Design review of the part built by this model. Coordinates are the model's own, in mm. A direction names the side the tool comes from. Coordinates: 2 decimals unless noted, no trailing zeros. Loops run counter-clockwise (first coordinate to the right, second up) from the corner with the lowest first, then second, coordinate; pieces in that order, holes last. Notation, with made-up numbers: (8, 25) -> (15, 25) arc R6 ccw to (15, 36) -> close; hole circle Ø2 at (71.25, -30). An arc over 180 degrees is marked (long way). Use one line per item in the form item = value. Start each with the question number.
1. For pin 1 (16.5 mm diameter, centred on x = 162.54, z = 38.1, fed in from -Y); pin 2 (4 mm diameter, centred on y = 28.5, z = 74, fed in from -X); pin 3 (2.5 mm diameter, centred on y = 36.5, z = 74.5, fed in from +X), all flat-tipped, find the tip position at first contact; note any pin that passes through.
2. Wall thickness on line 1 (Z direction, x = 19.05, y = 2.55); line 2 (X direction, y = 57, z = 25); line 3 (Y direction, x = 169.5, z = 46.5) (1 decimal): over which ranges is each line inside the solid? List them lowest first. Write a range as from..to.
3. Consider section B-B (y = 13.5). State the section outline as (x, z) points.
4. Consider section C-C (z = 25.4). State the section outline as (x, y) points (1 decimal).
5. Consider section D-D (x = 112). State the section outline as (y, z) points (1 decimal), then the cut area to 3 significant figures.
6. Machinability: for faces 1 (the face through (119, 30, 4.763)), 2 (the face through (14.292, 57.91, 25.609)), 3 (the face through (102.763, 30, 74)), 4 (the face through (135.793, 30, 2)), which of the approach directions +Z, -Z, +X, -X, +Y, -Y give a long, thin tool a straight path to every point of the face, cutting with its end or side? Answer none if there is none.
7. The part is to be moulded in two halves that separate along Y. For faces 5 (the face through (157.5, 57.91, 34.236)), 6 (the face through (100, 55.562, 38)), 7 (the face through (100, 60.325, 39)), say which applies: released by +Y, released by -Y, zero draft, split by the parting line, or undercut.
8. Consider section A-A (z = 38.1). State the section outline as (x, y) points (1 decimal), then the cut area to 3 significant figures.
from build123d import *

# Parameters (mm, degrees)
F0_W     = 203.2
F0_H     = 76.2
F0_R     = 4.7625
F0_R_2   = 6.35
F1_DEPTH = 60.325
F3_W     = 102.7627293737
F3_H     = 50.8
F4_DEPTH = 85.725
F5_W     = 50.8
F5_H     = 66.675
F6_DEPTH = 203.2
F7_W     = 67.4074530634
F7_H     = 50.8
F8_DEPTH = 76.2


with BuildPart() as f1:
    # F0 (on Front) → F1 (new body)
    with BuildSketch(Plane.XZ):
        with Locations((101.6, 38.1)):
            Rectangle(F0_W, F0_H)
        with Locations((19.05, 25.4)):
            Circle(F0_R, mode=Mode.SUBTRACT)
        with Locations((121.8779161572, 25.4)):
            Circle(F0_R, mode=Mode.SUBTRACT)
        with Locations((19.05, 50.8)):
            Circle(F0_R, mode=Mode.SUBTRACT)
        with Locations((121.8779161572, 50.8)):
            Circle(F0_R, mode=Mode.SUBTRACT)
        with Locations((162.5389580786, 38.1)):
            Circle(F0_R_2, mode=Mode.SUBTRACT)
    extrude(amount=-F1_DEPTH)

    # F3 (on offset) → F4 (cut)
    with BuildSketch(Plane.XY.offset(76.2)):
        with Locations((51.3813646869, 30.1625)):
            Rectangle(F3_W, F3_H)
    extrude(amount=-F4_DEPTH, mode=Mode.SUBTRACT)

    # F5 (on Right) → F6 (cut)
    with BuildSketch(Plane.YZ):
        with Locations((30.1625, 38.1)):
            Rectangle(F5_W, F5_H)
    extrude(amount=F6_DEPTH, mode=Mode.SUBTRACT)

    # F7 (on Top) → F8 (cut)
    with BuildSketch(Plane.XY):
        with Locations((169.4962734683, 30.1625)):
            Rectangle(F7_W, F7_H)
    extrude(amount=F8_DEPTH, mode=Mode.SUBTRACT)


solid = f1.part
Geometry check:
q1.pin_1 = 0
q1.pin_2 = 102.76
q1.pin_3 = 135.79
q2.line_1 = 0..20.64, 30.16..46.04, 55.56..76.2
q2.line_2 = 0..14.3, 23.8..117.13, 126.62..203.2
q2.line_3 = 0..4.8, 55.6..60.3
q3.outline = (102.76, 0) -> (135.79, 0) -> (135.79, 4.76) -> (102.76, 4.76) -> close; (102.76, 71.44) -> (135.79, 71.44) -> (135.79, 76.2) -> (102.76, 76.2) -> close
q4.outline = (0, 0) -> (14.3, 0) -> (14.3, 4.8) -> (0, 4.8) -> close; (0, 55.6) -> (14.3, 55.6) -> (14.3, 60.3) -> (0, 60.3) -> close; (23.8, 0) -> (117.1, 0) -> (117.1, 4.8) -> (23.8, 4.8) -> close; (23.8, 55.6) -> (117.1, 55.6) -> (117.1, 60.3) -> (23.8, 60.3) -> close; (126.6, 0) -> (203.2, 0) -> (203.2, 4.8) -> (126.6, 4.8) -> close; (126.6, 55.6) -> (203.2, 55.6) -> (203.2, 60.3) -> (126.6, 60.3) -> close
q5.outline = (0, 0) -> (60.3, 0) -> (60.3, 76.2) -> (0, 76.2) -> close; hole (4.8, 4.8) -> (55.6, 4.8) -> (55.6, 71.4) -> (4.8, 71.4) -> close
q5.area = 1,210 mm²
q6.face_1 = +X, -X
q6.face_2 = +Y, -Y
q6.face_3 = +Z, -Z, -X
q6.face_4 = +Z, -Z, +X
q7.face_5 = zero draft
q7.face_6 = undercut
q7.face_7 = released by +Y
q8.outline = (0, 0) -> (156.2, 0) -> (156.2, 4.8) -> (0, 4.8) -> close; (0, 55.6) -> (156.2, 55.6) -> (156.2, 60.3) -> (0, 60.3) -> close; (168.9, 0) -> (203.2, 0) -> (203.2, 4.8) -> (168.9, 4.8) -> close; (168.9, 55.6) -> (203.2, 55.6) -> (203.2, 60.3) -> (168.9, 60.3) -> close
q8.area = 1,810 mm²
